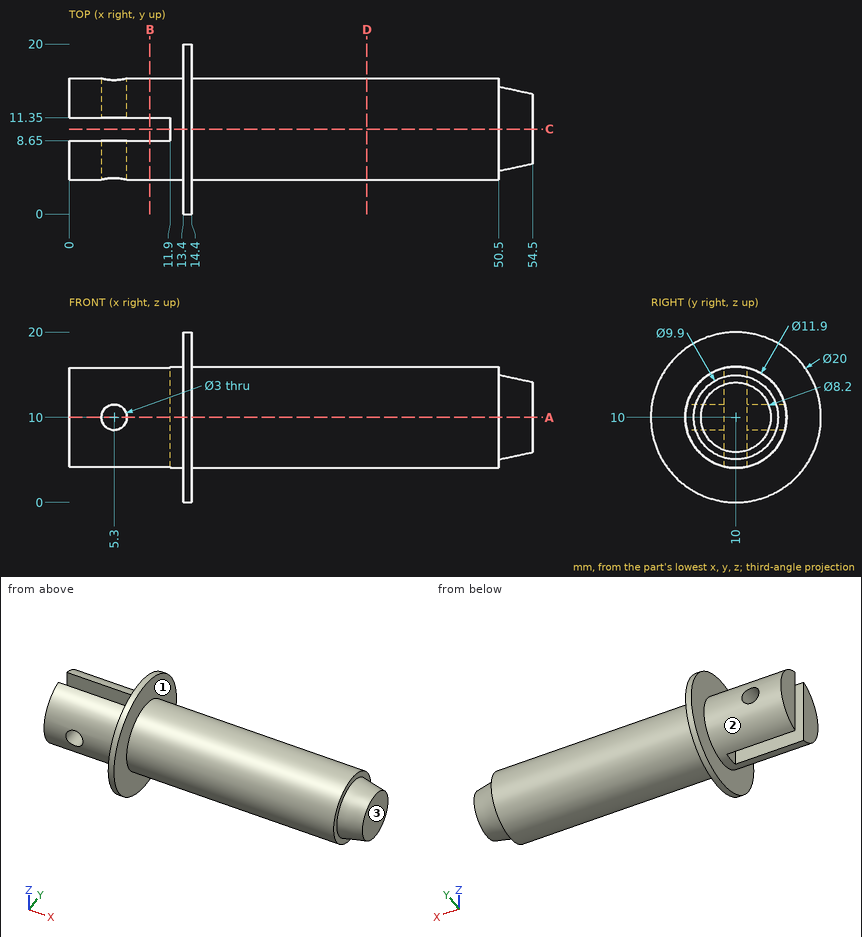
Print and shaded views of the part. All mm, measured from the part's lowest x, y and z. A direction names the side the tool comes from. Give positions to 0.01 mm unless a question says otherwise; leave off trailing zeros. Loops run counter-clockwise (first coordinate to the right, second up) from the corner with the lowest first, then second, coordinate; pieces in that order, holes last.
1) Saw through at C-C (y = 10). Write the cut outline in (x, z), plus the area to 3 significant figures.
2) Flat gauge pins, fed straight in: pin 1 Ø8 at (x, z) = (6.5, 13) entering from +Y; pin 2 Ø8 at (x, z) = (12, 16.5) entering from -Y; pin 3 Ø2.5 at (x, z) = (5.3, 10) entering from -Y; pin 4 Ø2 at (y, z) = (10, 6.5) entering from -X. Where does each tip first touch, or does it go through?
3) Tool access for the marked faces 1, 2 and 3: list every direction of +Z, -Z, +X, -X, +Y, -Y with a clear straight run to the whole face (end or side of a thin tool).
4) Saw through at A-A (z = 10). Write the cut outline in (x, y), plus the area to 3 significant figures.
5) Saw through at B-B (x = 9.5). Write the cut outline in (y, z), plus the area to 3 significant figures.
6) Wall check: line 1 (X direction, y = 13.15, z = 10); line 2 (X direction, y = 18, z = 10); line 3 (X direction, y = 13.75, z = 5.75). Give the ranges that are in metal, low to high.
7) Saw through at D-D (x = 35). Write the cut outline in (y, z), plus the area to 3 significant figures.
Answer block:
1. outline: (11.9, 4.05) - (13.4, 4.05) - (13.4, 0) - (14.4, 0) - (14.4, 4.05) - (50.5, 4.05) - (50.5, 5.05) - (54.5, 5.9) - (54.5, 14.1) - (50.5, 14.95) - (50.5, 15.95) - (14.4, 15.95) - (14.4, 20) - (13.4, 20) - (13.4, 15.95) - (11.9, 15.95) - close
1. area: 504 mm2
2. pin 1: stops at y = 15.95
2. pin 2: stops at y = 0.39
2. pin 3: passes through
2. pin 4: stops at x = 11.9
3. face 1: +X
3. face 2: -X
3. face 3: +Z, -Z, +X, +Y, -Y
4. outline: (0, 4.05) - (3.8, 4.05) - (3.8, 8.65) - (0, 8.65) - close; (0, 11.35) - (3.8, 11.35) - (3.8, 15.95) - (0, 15.95) - close; (6.8, 4.05) - (13.4, 4.05) - (13.4, 0) - (14.4, 0) - (14.4, 4.05) - (50.5, 4.05) - (50.5, 5.05) - (54.5, 5.9) - (54.5, 14.1) - (50.5, 14.95) - (50.5, 15.95) - (14.4, 15.95) - (14.4, 20) - (13.4, 20) - (13.4, 15.95) - (6.8, 15.95) - (6.8, 11.35) - (11.9, 11.35) - (11.9, 8.65) - (6.8, 8.65) - close
4. area: 586 mm2
5. outline: (8.65, 4.21) - (8.65, 15.79) arc R5.95 ccw to start; (11.35, 4.21) arc R5.95 ccw to (11.35, 15.79) - close
5. area: 79.4 mm2
6. line 1: x = 0 to 3.8, 6.8 to 54.5
6. line 2: x = 13.4 to 14.4
6. line 3: x = 0 to 50.5
7. outline: circle Ø11.9 at (10, 10)
7. area: 111 mm2
